CAD build for the part. Positions are in the model's coordinates, mm. A direction names the side the tool comes from. Give positions to 0.01 mm unless a question says otherwise; leave off trailing zeros. Write each loop counter-clockwise with the first axis right and the second up, starting at its lowest first coordinate (ties: lowest second). Pieces come first, ordered by that corner, then holes. Notation, with made-up numbers: (49.25, -28.5) -> (71.25, -28.5) arc R22 ccw to (71.25, 6.5) -> close; hole circle Ø5 at (14, 29.25). An arc over 180 degrees is marked (long way). Answer as a JSON object with one key per item and string values.
```python
from build123d import *

# Parameters (mm, degrees)
F1_DEPTH = 6.35
F2_R     = 3.175
F3_R     = 6.35


with BuildPart() as f1:
    # F0 (on Front) → F1 (new body, symmetric)
    with BuildSketch(Plane.XZ):
        Polygon((15, 0), (0, 0), (-15, 0), (-15, 20), (-18.175, 20), (-18.175, -3.175), (0, -3.175), (18.175, -3.175), (18.175, 20), (15, 20), align=None)
    extrude(amount=F1_DEPTH, both=True)

    # F2
    f2_edges = [f1.edges().sort_by_distance(p)[0] for p in [
        (15, 0, 0),
        (-15, 0, 0),
    ]]
    fillet(f2_edges, radius=F2_R)

    # F3
    f3_edges = [f1.edges().sort_by_distance(p)[0] for p in [
        (-18.175, 0, -3.175),
        (18.175, 0, -3.175),
    ]]
    fillet(f3_edges, radius=F3_R)


solid = f1.part
```
1) 3-axis set-ups, long thin cutter, end or side, ignore diameter. For faces 1 (the cylindrical face through (14.05, 0.09, 0.91)), 2 (the flat face through (-18.175, 0, 12)): which of +Z, -Z, +X, -X, +Y, -Y reach the whole face in a straight line?
Model answer:
{"face 1": "+Z, +Y, -Y", "face 2": "+Z, -Z, -X, +Y, -Y"}
2) Slice it at C-C (x = -4.5). List the corners of the cut face in (y, z) (3 decimals), then the cut area to 3 significant figures.
Model answer:
{"outline": "(-6.35, -3.175) -> (6.35, -3.175) -> (6.35, 0) -> (-6.35, 0) -> close", "area": "40.3 mm2"}
3) Slice it at B-B (y = 0). List the corners of the cut face in (x, z) (3 decimals), then the cut area to 3 significant figures.
Model answer:
{"outline": "(-18.175, 3.175) arc R6.35 ccw to (-11.825, -3.175) -> (11.825, -3.175) arc R6.35 ccw to (18.175, 3.175) -> (18.175, 20) -> (15, 20) -> (15, 3.175) arc R3.175 cw to (11.825, 0) -> (-11.825, 0) arc R3.175 cw to (-15, 3.175) -> (-15, 20) -> (-18.175, 20) -> close", "area": "229 mm2"}
4) Slice it at A-A (z = 18.25). List the corners of the cut face in (x, y) (3 decimals).
Model answer:
{"outline": "(-18.175, -6.35) -> (-15, -6.35) -> (-15, 6.35) -> (-18.175, 6.35) -> close; (15, -6.35) -> (18.175, -6.35) -> (18.175, 6.35) -> (15, 6.35) -> close"}
5) Mould opens along X. For faces 3 (the flat face through (-15, 0, 11)), 4 (the flat face through (17, 0, 20)), 5 (the cylindrical face through (16.36, -0.09, -1.27)) say: released by +X, released by -X, zero draft, split by the parting line, or undercut.
Model answer:
{"face 3": "undercut", "face 4": "zero draft", "face 5": "released by +X"}
6) Slice it at D-D (z = 2.5). List the corners of the cut face in (x, y).
Model answer:
{"outline": "(-18.14, -6.35) -> (-14.93, -6.35) -> (-14.93, 6.35) -> (-18.14, 6.35) -> close; (14.93, -6.35) -> (18.14, -6.35) -> (18.14, 6.35) -> (14.93, 6.35) -> close"}
7) Pin check, flat tips, straight feed: pin 1 (6 mm diameter, centred on x = 10.5, y = -2, fed in from +Z); pin 2 (12 mm diameter, centred on x = -5.5, z = 14, fed in from +Y); pin 3 (4 mm diameter, centred on x = 8, y = 4.5, fed in from +Z). Stop position of each tip, or through.
Model answer:
{"pin 1": "stops at z = 0.48", "pin 2": "passes through", "pin 3": "stops at z = 0"}
8) Wall check: probe 1 along X at (y, z) = (1.75, 12) (3 decimals); probe 2 along Z at (x, y) = (7, 1) (3 decimals); probe 3 along Z at (x, y) = (-14, 1.5). Give the ranges that are in metal, low to high.
Model answer:
{"probe 1": "x = -18.175 to -15, 15 to 18.175", "probe 2": "z = -3.175 to 0", "probe 3": "z = -2.79 to 0.86"}
